from build123d import *

# Parameters (mm, degrees)
F1_DEPTH = 127


with BuildPart() as f1:
    # F0 (on Right) → F1 (new body, symmetric)
    with BuildSketch(Plane.YZ):
        Polygon((-154.398493, 87.090496), (-115.932986, 142.508402), (-49.40985, 135.687735), (-45.471936, 142.508402), (-80.702461, 203.529462), (-151.163511, 203.529462), (-186.394036, 142.508402), align=None)
    extrude(amount=F1_DEPTH, both=True)


solid = f1.part
Geometry: final body of the model. Coordinates: model frame, mm. A direction names the side the tool comes from. Coordinates: 2 decimals unless noted, no trailing zeros. Order: outer loops, then holes, each group sorted by start corner. A loop starts at its lowest first (then second) coordinate and runs counter-clockwise, first axis right, second up. Notation, with made-up numbers: M 54,75 L 65,75 A33 cw 65,112 Z; hole C 43.25,46 d3. An arc over 180 degrees is marked long. One line per question, with ' | ' between items. Start each with the question number.
Item 1: Cut plane C-C, the plane z = 115. Return the cut outline in (x, y), then the cut area to 3 significant figures.
Item 2: Cut plane B-B, the plane y = -72. Return the cut outline in (x, z), then the cut area to 3 significant figures.
Item 3: Set-up query: faces 1 (the flat face through (1.778, -83.137, 139.146)), 2 (the flat face through (1.78, -168.53, 173.45)). Return all of +Z, -Z, +X, -X, +Y, -Y with unobstructed straight access to the full face (end or side cutting, diameter ignored); none if empty.
Item 4: Cut plane A-A, the plane x = 68. Return the cut outline in (y, z), then the cut area to 3 significant figures.
Item 5: Ray query, probe 1 along Y at (x, z) = (52, 101.5); probe 2 along Z at (x, y) = (-68.5, -155.5); probe 3 along Y at (x, z) = (-107, 123). Return the intervals inside material, ascending. Write a range as [from, to].
Item 6: Pin query (flat end, axial travel): pin 1 Ø12 at (x, y) = (72, -104.5) entering from -Z; pin 2 Ø6 at (x, y) = (74, -168) entering from -Z; pin 3 Ø3 at (x, y) = (98, -152) entering from -Z (3 decimals). Return the tip coordinate at first contact, or that it passes through.
A:
1) outline: M -127,-170.51 L 127,-170.51 L 127,-135.03 L -127,-135.03 Z | area: 9,010 mm2
2) outline: M -127,138 L 127,138 L 127,188.46 L -127,188.46 Z | area: 12,800 mm2
3) face 1: -Z, +X, -X | face 2: +Z, +X, -X, -Y
4) outline: M -186.39,142.51 L -154.4,87.09 L -115.93,142.51 L -49.41,135.69 L -45.47,142.51 L -80.7,203.53 L -151.16,203.53 Z | area: 8,640 mm2
5) probe 1: y = [-162.72, -144.4] | probe 2: z = [89, 196.02] | probe 3: y = [-175.13, -129.47]
6) pin 1: stops at z = 140.72 | pin 2: stops at z = 105.45 | pin 3: stops at z = 88.385
